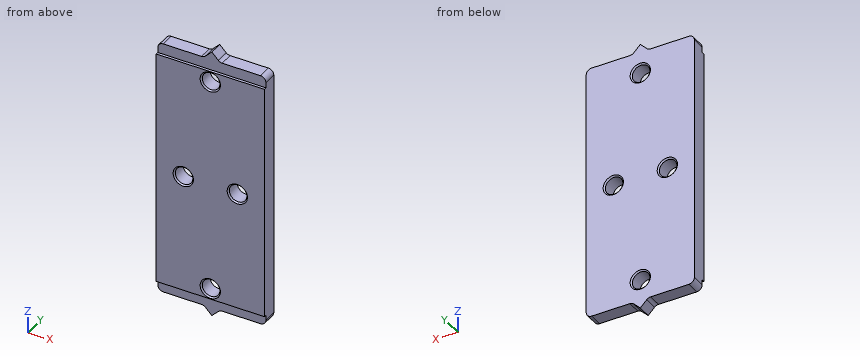
Autodesk Inventor part; units mm, degrees
ref_plane "XZ Plane" through (0, 0, 0) normal (0, 1, 0) x (-1, 0, 0)
sketch "Skizze1" plane through (0, 0, 0) normal (0, 0, 1) x (1, 0, 0)
  line L0 (-20, 3) -> (20, 3)
  line L1 (20, 3) -> (20, -3)
  line L2 (20, -3) -> (-20, -3)
  line L3 (-20, -3) -> (-20, 3)
  line L4 (-20, 3) -> (20, -3) construction
  line L5 (20, 3) -> (-20, -3) construction
  point P0 (0, 0)
  dimension "d0" = 6
  dimension "d2" = 40
extrude "Extrusion1" add sketch "Skizze1" along normal mid plane 96
sketch "Skizze3" plane through (-20, 3, 48) normal (0, 1, 0) x (1, 0, 0)
  line L0 (0, 96) -> (0, 0)
  line L1 (40, 0) -> (0, 0)
  line L2 (40, 96) -> (40, 0)
  line L3 (0, 96) -> (40, 96)
  point P0 (20, 48)
  point P1 (10, 48)
  point P2 (30, 48)
  point P3 (0, 48)
  dimension "d5" = 10
  dimension "d6" = 10
hole "Bohrung1" at (-10, 3, 0) at (10, 3, 0) direction (0, -1, 0) diameter 6.5 end through all
sketch "Skizze4" plane through (-20, 3, 48) normal (0, 1, 0) x (1, 0, 0)
  circle A0 centre (30, 48) radius 3.25
  circle A1 centre (10, 48) radius 3.25
  line L0 (0, 96) -> (0, 0)
  line L1 (40, 0) -> (0, 0)
  line L2 (40, 96) -> (40, 0)
  line L3 (0, 96) -> (40, 96)
  point P0 (20, 48)
  point P1 (20, 8)
  point P2 (20, 88)
  dimension "d14" = 40
  dimension "d15" = 40
hole "Bohrung2" at (0, 3, 40) at (0, 3, -40) direction (0, -1, 0) diameter 6.5 end through all
sketch "Skizze5" plane through (-20, 3, 48) normal (0, 1, 0) x (1, 0, 0)
  circle A0 centre (20, 88) radius 3.25
  circle A1 centre (20, 8) radius 3.25
  circle A2 centre (30, 48) radius 3.25
  circle A3 centre (10, 48) radius 3.25
  line L0 (0, 96) -> (0, 0)
  line L1 (40, 0) -> (0, 0)
  line L2 (40, 96) -> (40, 0)
  line L3 (0, 96) -> (40, 96)
  line L4 (20, 115.8) -> (20, -22.8)
  line L5 (40, 0) -> (0, 0)
  line L6 (20, -3) -> (23, 0)
  line L7 (20, -3) -> (17, 0)
  line L8 (0, 0) -> (40, 0)
  point P0 (20, 48)
  dimension "d29" = 6
  dimension "d30" = 3
  dimension "d31" = 45
extrude "Extrusion2" add sketch "Skizze5" against normal up to surface (6 mm away) contours L4 L7 L1 | L1 L6 L4
mirror "Spiegeln1" about plane through (0, 0, 0) normal (1, 0, 0) of "Extrusion2"
mirror "Spiegeln2" about plane through (0, 0, 0) normal (0, 0, 1) of "Extrusion2", "Spiegeln1"
fillet "Rundung1" radius 2 4 edges at (-20, 0, 48) (20, 0, 48) (-20, 0, -48) (20, 0, -48)
fillet "Rundung2" radius 2 4 edges at (-3, 0, 48) (3, 0, 48) (-3, 0, -48) (3, 0, -48)
sketch "Skizze6" plane through (20, -3, -46) normal (0, -1, 0) x (1, 0, 0)
  circle A0 centre (-20, 6) radius 3.25
  circle A1 centre (-20, 86) radius 3.25
  circle A2 centre (-10, 46) radius 3.25
  circle A3 centre (-30, 46) radius 3.25
  arc A4 (-2, -2) -> (0, 0) centre (-2, 0) ccw
  line L0 (0, 0) -> (0, 92)
  arc A5 (0, 92) -> (-2, 94) centre (-2, 92) ccw
  line L1 (-16.1716, 94) -> (-2, 94)
  arc A6 (-17.5858, 94.5858) -> (-16.1716, 94) centre (-16.1716, 96) ccw
  line L2 (-20, 97) -> (-17.5858, 94.5858)
  line L3 (-22.4142, 94.5858) -> (-20, 97)
  arc A7 (-23.8284, 94) -> (-22.4142, 94.5858) centre (-23.8284, 96) ccw
  line L4 (-38, 94) -> (-23.8284, 94)
  arc A8 (-38, 94) -> (-40, 92) centre (-38, 92) ccw
  line L5 (-40, 92) -> (-40, 0)
  arc A9 (-40, 0) -> (-38, -2) centre (-38, 0) ccw
  line L6 (-23.8284, -2) -> (-38, -2)
  arc A10 (-22.4142, -2.5858) -> (-23.8284, -2) centre (-23.8284, -4) ccw
  line L7 (-22.4142, -2.5858) -> (-20, -5)
  line L8 (-20, -5) -> (-17.5858, -2.5858)
  arc A11 (-16.1716, -2) -> (-17.5858, -2.5858) centre (-16.1716, -4) ccw
  line L9 (-2, -2) -> (-16.1716, -2)
  line L10 (-59.3165, 111.9132) -> (18.0456, 111.9132)
  line L11 (18.0456, 111.9132) -> (18.0456, 90)
  line L12 (18.0456, 90) -> (-59.3165, 90)
  line L13 (-59.3165, 90) -> (-59.3165, 111.9132)
  line L14 (-80.9876, 2) -> (21.6776, 2)
  line L15 (21.6776, 2) -> (21.6776, -24.7559)
  line L16 (21.6776, -24.7559) -> (-80.9876, -24.7559)
  line L17 (-80.9876, -24.7559) -> (-80.9876, 2)
  point P0 (-20, 46)
  point P1 (-40, 2)
  point P2 (0, 2)
  dimension "d34" = 4
  dimension "d35" = 4
  dimension "d36" = 77.3621
  dimension "d37" = 21.9132
  dimension "d38" = 102.6652
  dimension "d39" = 26.7559
extrude "Extrusion3" cut sketch "Skizze6" against normal blind 1 contours L9 A11 L8 L7 A10 L6 A9 L5 L14 L0 A4 | A4 L0 L14 L15 L16 L17 L5 A9 L6 A10 L7 L8 A11 L9 | L12 L5 A8 L4 A7 L3 L2 A6 L1 A5 L0 | L0 A5 L1 A6 L2 L3 A7 L4 A8 L5 L12 L13 L10 L11
chamfer "Fasen1" distance 0.5 angle 45 4 edges at (-10, -3, -3.25) (-10, 3, -3.25) (10, -3, -3.25) (10, 3, -3.25)
chamfer "Fasen2" distance 0.5 angle 45 2 edges at (0, -3, 36.75) (0, 3, 36.75)
chamfer "Fasen3" distance 0.5 angle 45 2 edges at (0, -3, -43.25) (0, 3, -43.25)
properties part number "Klemmplatte"
Build history of the part. All positions in model axes, mm. Give positions to 0.01 mm unless a question says otherwise; leave off trailing zeros. Order: outer loops, then holes, each group sorted by start corner. A loop starts at its lowest first (then second) coordinate and runs counter-clockwise, first axis right, second up. Notation, with made-up numbers: M -1,30.25 L 44,30.25 A34 ccw 44,60.25 Z; hole C -23,52 d9. An arc over 180 degrees is marked long. Write item = value, one per line. Start each with the question number.
(1) Slice it at C-C on x = -17. Write the cut outline in (y, z).
(2) Pin check, flat tips, straight feed: pin 1 Ø7.5 at (x, z) = (6, 48) entering from -Y; pin 2 Ø4 at (x, z) = (10, 0) entering from +Y; pin 3 Ø1.1 at (x, y) = (8.5, -2.5) entering from +Z; pin 4 Ø2.5 at (x, y) = (11, 1) entering from -Z. Stop position of each tip, or through.
(3) Probe L1, parallel to X at y = -1.05, z = 0; L2, parallel to Z at x = 0, y = -0.45; L3, parallel to X at y = 2.5, z = 40. List the from-to ranges inside material, lowest first. Write a range as [from, to].
(4) Slice it at A-A on z = 0. Write the cut outline in (x, y), plus the area to 3 significant figures.
(5) Slice it at D-D on z = 40. Write the cut outline in (x, y), plus the area to 4 significant figures.
(6) Slice it at B-B on y = -0.4. Write the cut outline in (x, z).
Responses:
q1.outline = M -3,-44 L -2,-44 L -2,-48 L 3,-48 L 3,48 L -2,48 L -2,44 L -3,44 Z
q2.pin_1 = -2
q2.pin_2 = through
q2.pin_3 = 48
q2.pin_4 = -48
q3.L1 = [-20, -13.25], [-6.75, 6.75], [13.25, 20]
q3.L2 = [-51, -43.25], [-36.75, 36.75], [43.25, 51]
q3.L3 = [-20, -3.25], [3.25, 20]
q4.outline = M -20,-3 L -13.75,-3 L -13.25,-2.5 L -13.25,2.5 L -13.75,3 L -20,3 Z; M -6.75,-2.5 L -6.25,-3 L 6.25,-3 L 6.75,-2.5 L 6.75,2.5 L 6.25,3 L -6.25,3 L -6.75,2.5 Z; M 13.25,-2.5 L 13.75,-3 L 20,-3 L 20,3 L 13.75,3 L 13.25,2.5 Z
q4.area = 161 mm2
q5.outline = M -20,-3 L -3.75,-3 L -3.25,-2.5 L -3.25,2.5 L -3.75,3 L -20,3 Z; M 3.25,-2.5 L 3.75,-3 L 20,-3 L 20,3 L 3.75,3 L 3.25,2.5 Z
q5.area = 200.5 mm2
q6.outline = M -20,-46 A2 ccw -18,-48 L -3.83,-48 A2 cw -2.41,-48.59 L 0,-51 L 2.41,-48.59 A2 cw 3.83,-48 L 18,-48 A2 ccw 20,-46 L 20,46 A2 ccw 18,48 L 3.83,48 A2 cw 2.41,48.59 L 0,51 L -2.41,48.59 A2 cw -3.83,48 L -18,48 A2 ccw -20,46 Z; hole C -10,0 d6.5; hole C 0,-40 d6.5; hole C 0,40 d6.5; hole C 10,0 d6.5
